Source: CAD feature listing. Evaluate the final solid. Frame: model axes, mm. Coordinates: 2 decimals unless noted, no trailing zeros. Order: outer loops, then holes, each group sorted by start corner. A loop starts at its lowest first (then second) coordinate and runs counter-clockwise, first axis right, second up. Notation, with made-up numbers: (58, -3.75) -> (97, -3.75) arc R19 ccw to (97, 7.25) -> close; hole circle Ø3 at (24, 46). An arc over 180 degrees is marked (long way). Put each result on its own line as item: value.
from build123d import *

# Parameters (mm, degrees)
SKETCH2_R           = 8
SKETCH2_R_2         = 4
BOSS_EXTRUDE1_DEPTH = 2.5
SKETCH3_R           = 9
BOSS_EXTRUDE3_DEPTH = 1
SKETCH5_R           = 4
CUT_EXTRUDE1_DEPTH  = 6


with BuildPart() as part:
    # Sketch2 → Boss-Extrude1 (new body, symmetric)
    with BuildSketch(Plane(origin=(0, 0, 0), x_dir=(1, 0, 0), z_dir=(0, 1, 0))):
        Circle(SKETCH2_R)
        Circle(SKETCH2_R_2, mode=Mode.SUBTRACT)
    extrude(amount=BOSS_EXTRUDE1_DEPTH, both=True)

    # Sketch3 → Boss-Extrude3 (add)
    with BuildSketch(Plane(origin=(0, 2.5, 0), x_dir=(1, 0, 0), z_dir=(0, 1, 0))):
        Circle(SKETCH3_R)
    extrude(amount=-BOSS_EXTRUDE3_DEPTH)

    # Sketch5 → Cut-Extrude1 (cut, through all)
    with BuildSketch(Plane.XZ.offset(2.5)):
        Circle(SKETCH5_R)
    extrude(amount=-CUT_EXTRUDE1_DEPTH, mode=Mode.SUBTRACT)


solid = part.part
1. Cut plane A-A on x = 0. Output: boundary loops of the cut face in (y, z).
Numbers:
outline: (-2.5, -8) -> (1.5, -8) -> (1.5, -9) -> (2.5, -9) -> (2.5, -4) -> (-2.5, -4) -> close; (-2.5, 4) -> (2.5, 4) -> (2.5, 9) -> (1.5, 9) -> (1.5, 8) -> (-2.5, 8) -> close
2. Pull-direction query (Z, two-part tool) for faces 1 (the flat face through (4, 2.5, 2)), 2 (the cylindrical face through (-0.867, -0.035, -3.905)), 3 (the cylindrical face through (-1.73, -0.47, 7.81)); classes: pulls with the +Z half, pulls with the -Z half, needs draft (parallel to the pull), parting line crosses it, or undercut.
Numbers:
face 1: needs draft
face 2: undercut
face 3: parting line crosses it
3. Cut plane B-B on z = 0. Output: boundary loops of the cut face in (x, y).
Numbers:
outline: (-9, 1.5) -> (-8, 1.5) -> (-8, -2.5) -> (-4, -2.5) -> (-4, 2.5) -> (-9, 2.5) -> close; (4, -2.5) -> (8, -2.5) -> (8, 1.5) -> (9, 1.5) -> (9, 2.5) -> (4, 2.5) -> close
4. Cut plane C-C on y = -0.7. Output: boundary loops of the cut face in (x, z).
Numbers:
outline: circle Ø16 at (0, 0); hole circle Ø8 at (0, 0)
5. First-contact query: pin 1 (3 mm diameter, centred on y = -2, z = -6.5, fed in from -X) (3 decimals); pin 2 (1.5 mm diameter, centred on x = -3.5, y = -1, fed in from -Z); pin 3 (6.5 mm diameter, centred on x = 0, z = 0, fed in from +Y) (3 decimals). Flat tips, straight axial feed; report the tip coordinate or a pass-through.
Numbers:
pin 1: stops at x = -6.245
pin 2: stops at z = -7.51
pin 3: passes through
6. Cut plane D-D on z = -6. Output: boundary loops of the cut face in (x, y), plus the area to 3 significant figures.
Numbers:
outline: (-6.71, 1.5) -> (-5.29, 1.5) -> (-5.29, -2.5) -> (5.29, -2.5) -> (5.29, 1.5) -> (6.71, 1.5) -> (6.71, 2.5) -> (-6.71, 2.5) -> close
area: 55.7 mm2
7. Ray query, line 1 along X through (y, z) = (1.4, 0); line 2 along X through (y, z) = (-2.15, 1.5). Return the intervals inside material, ascending.
Numbers:
line 1: x = -8 to -4, 4 to 8
line 2: x = -7.86 to -3.71, 3.71 to 7.86
